Solid Edge part; units mm, degrees
sketch "Sketch1" plane through (0, 0, 0) normal (0, -1, 0) x (1, 0, 0)
  line L0 (1.1931, 20) -> (12, 20)
  arc A0 (1.1931, 20) -> (-1.2404, 19.3679) centre (1.1931, 15) ccw
  line L1 (-10.2148, 14.3679) -> (-1.2404, 19.3679)
  arc A1 (-10.2148, 14.3679) -> (-10.2148, 5.6321) centre (-7.7813, 10) ccw
  line L2 (-1.2404, 0.6321) -> (-10.2148, 5.6321)
  arc A2 (-1.2404, 0.6321) -> (1.1931, 0) centre (1.1931, 5) ccw
  line L3 (12, 0) -> (1.1931, 0)
  line L4 (12, 2) -> (12, 0)
  line L5 (12, 2) -> (1.1931, 2)
  arc A3 (1.1931, 2) -> (-0.267, 2.3793) centre (1.1931, 5) cw
  line L6 (-0.267, 2.3793) -> (-9.2414, 7.3793)
  arc A4 (-9.2414, 7.3793) -> (-9.2414, 12.6207) centre (-7.7813, 10) cw
  line L7 (-9.2414, 12.6207) -> (-0.267, 17.6207)
  arc A5 (-0.267, 17.6207) -> (1.1931, 18) centre (1.1931, 15) cw
  line L8 (1.1931, 18) -> (12, 18)
  line L9 (12, 20) -> (12, 18)
extrude "Protrusion1" add sketch "Sketch1" along normal mid plane 12
sketch "Sketch2" plane through (6.5966, 0, 20) normal (0, 0, 1) x (1, 0, 0)
  circle A0 centre (0, 0) radius 2.2
extrude "Cutout1" cut sketch "Sketch2" against normal through all
Source: CAD feature listing. Evaluate the final solid. Frame: model axes, mm. A direction names the side the tool comes from. Coordinates: 2 decimals unless noted, no trailing zeros. Loops run counter-clockwise (first coordinate to the right, second up) from the corner with the lowest first, then second, coordinate; pieces in that order, holes last. Notation, with made-up numbers: M -29,83 L 0,83 A14 cw 0,98 Z; hole C 35.25,43 d4. An arc over 180 degrees is marked long. Answer in a Markdown table with one row per item.
Q1. Section A-A on x = 9.25. Return the cut outline in (y, z), plus the area to 3 significant figures.
Answers below:
| item | result |
|---|---|
| outline | M -6,0 L 6,0 L 6,2 L -6,2 Z; M -6,18 L 6,18 L 6,20 L -6,20 Z |
| area | 48.0 mm^2 |
Q2. First-contact query: pin 1 (6 mm diameter, centred on y = 0.5, z = 10, fed in from +X); pin 2 (3 mm diameter, centred on x = -1, y = 3, fed in from -Z); pin 3 (1 mm diameter, centred on y = 4, z = 13.5, fed in from +X). Flat tips, straight axial feed; report the tip coordinate or a pass-through.
Answers below:
| item | result |
|---|---|
| pin 1 | stops at x = -8.56 |
| pin 2 | stops at z = 0.05 |
| pin 3 | stops at x = -6.77 |
Q3. Section B-B on y = 0. Return the cut outline in (x, z), plus the area to 3 significant figures.
Answers below:
| item | result |
|---|---|
| outline | M -10.21,5.63 L -1.24,0.63 A5 ccw 1.19,0 L 4.4,0 L 4.4,2 L 1.19,2 A3 cw -0.27,2.38 L -9.24,7.38 A3 cw -9.24,12.62 L -0.27,17.62 A3 cw 1.19,18 L 4.4,18 L 4.4,20 L 1.19,20 A5 ccw -1.24,19.37 L -10.21,14.37 A5 ccw Z; M 8.8,0 L 12,0 L 12,2 L 8.8,2 Z; M 8.8,18 L 12,18 L 12,20 L 8.8,20 Z |
| area | 91.9 mm^2 |
Q4. Section C-C on x = -3.5. Return the cut outline in (y, z).
Answers below:
| item | result |
|---|---|
| outline | M -6,1.89 L 6,1.89 L 6,4.18 L -6,4.18 Z; M -6,15.82 L 6,15.82 L 6,18.11 L -6,18.11 Z |
Q5. Set-up query: faces 5 (the cylindrical face through (-0.047, 0.084, 0.156)), 6 (the cylindrical face through (0.43, 0.08, 17.9)). Return all of +Z, -Z, +X, -X, +Y, -Y with unobstructed straight access to the full face (end or side cutting, diameter ignored); none if empty.
Answers below:
| item | result |
|---|---|
| face 5 | -Z, -X, +Y, -Y |
| face 6 | +X, +Y, -Y |
Q6. Ray query, probe 1 along Z at (x, y) = (9.75, 0); probe 2 along Z at (x, y) = (-2, 3); probe 3 along X at (y, z) = (1.25, 19). Return the intervals inside material, ascending. Write a range as from..to.
Answers below:
| item | result |
|---|---|
| probe 1 | z = 0..2, 18..20 |
| probe 2 | z = 1.06..3.34, 16.66..18.94 |
| probe 3 | x = -1.9..4.79, 8.41..12 |
Q7. Draft query along Y for faces 1 (the cylindrical face through (6.31, 2.18, 1.01)), 2 (the cylindrical face through (-0.081, 0.084, 19.835)), 3 (the flat face through (-4, 6, 4)), 4 (the flat face through (-4, -6, 4)). Return one class per face: pulls with the +Y half, pulls with the -Y half, needs draft (parallel to the pull), parting line crosses it, or undercut.
Answers below:
| item | result |
|---|---|
| face 1 | undercut |
| face 2 | needs draft |
| face 3 | pulls with the +Y half |
| face 4 | pulls with the -Y half |
Q8. Section D-D on z = 10.75. Return the cut outline in (x, y).
Answers below:
| item | result |
|---|---|
| outline | M -12.72,-6 L -10.69,-6 L -10.69,6 L -12.72,6 Z |
